Here's how the part is built. I have some questions about the finished solid (model axes, mm). A direction names the side the tool comes from. Give positions to 0.01 mm unless a question says otherwise; leave off trailing zeros. Write each loop counter-clockwise with the first axis right and the second up, starting at its lowest first coordinate (ties: lowest second). Pieces come first, ordered by that corner, then holes. Notation, with made-up numbers: (-6.5, 71) -> (10.5, 71) arc R11 cw to (10.5, 84) -> close; hole circle Ø11 at (9, -4.75). An arc over 180 degrees is marked (long way). Use CSV: the item, a comma, the result in double quotes. Start each with the question number.
(1) If we mould it in two halves opening along X, with no side actions, what happens to faces 1 (the flat face through (-1.5, 4.166, -1.5)), 2 (the flat face through (0, 2, -1.786)), 3 (the cylindrical face through (1.987, -6.439, 0.626))? For each: pulls with the +X half, pulls with the -X half, needs draft (parallel to the pull), parting line crosses it, or undercut.
(2) I need wall thicknesses on L1, parallel to Z at x = 0, y = 2; L2, parallel to Y at x = -2, z = -2.25; L3, parallel to X at y = 1, z = -0.5. Which ranges of each line are inside material? Lowest first, please. Write a range as [from, to].
(3) Suppose I cut it at D-D on y = -1.75. List the corners of the cut face in (x, z) for me.
(4) Suppose I cut it at C-C on x = 0. List the corners of the cut face in (y, z) for me, plus the area to 3 significant figures.
(5) For pin 1 Ø4 at (x, z) = (0.5, 1.5) entering from +Y; pin 2 Ø1 at (y, z) = (-9.5, 1) entering from -X; pin 3 Ø1.8 at (x, z) = (-0.5, 0) entering from +Y; pin 4 Ø1 at (x, y) = (-0.5, -3) entering from +Z, each with a flat end and sliding along its axis, tell me the tip position at first contact or that it passes through.
(6) Suppose I cut it at B-B on z = -1.25. List the corners of the cut face in (x, y) for me.
(7) Suppose I cut it at A-A on y = 2.25. List the corners of the cut face in (x, z) for me.
(8) Which directions (+Z, -Z, +X, -X, +Y, -Y) give clear straight access to the entire face, cutting with the end or side of a thin tool? Please do faces 4 (the flat face through (-0.05, 0, -2.24)), 5 (the cylindrical face through (-0.74, 2.05, -3.35)), 6 (the flat face through (-1.554, 2.405, 0.88)).
from build123d import *

# Parameters (mm, degrees)
CUT_EXTRUDE1_DEPTH = 3.571875


with BuildPart() as part:
    # profiile → Base-Revolve (revolve)
    with BuildSketch(Plane.XY):
        Polygon((0, 4.1656), (3.429, 4.1656), (3.429, 0), (2.0828, 0), (2.0828, -12.7), (0, -12.7), align=None)
    revolve(axis=Axis((0, 9.907210965, 0), (0, -1, 0)))

    # Sketch1 → Cut-Extrude1 (cut)
    with BuildSketch(Plane(origin=(0, 4.1656, 0), x_dir=(1, 0, 0), z_dir=(0, 1, 0))):
        Polygon((2.062222993, 0), (1.031111496, 1.7859375), (-1.031111496, 1.7859375), (-2.062222993, 0), (-1.031111496, -1.7859375), (1.031111496, -1.7859375), align=None)
    extrude(amount=-CUT_EXTRUDE1_DEPTH, mode=Mode.SUBTRACT)


solid = part.part
Geometry says:
1,face 1,"needs draft"
1,face 2,"undercut"
1,face 3,"parting line crosses it"
2,L1,"[-3.43, -1.79], [1.79, 3.43]"
2,L2,"[0, 4.17]"
2,L3,"[-3.39, -1.77], [1.77, 3.39]"
3,outline,"circle Ø4.17 at (0, 0)"
4,outline,"(-12.7, -2.08) -> (0, -2.08) -> (0, -3.43) -> (4.17, -3.43) -> (4.17, -1.79) -> (0.59, -1.79) -> (0.59, 1.79) -> (4.17, 1.79) -> (4.17, 3.43) -> (0, 3.43) -> (0, 2.08) -> (-12.7, 2.08) -> close"
4,area,"68.7 mm²"
5,pin 1,"y = 4.17"
5,pin 2,"x = -2.02"
5,pin 3,"y = 0.59"
5,pin 4,"z = 2.08"
6,outline,"(-3.19, 0) -> (-1.67, 0) -> (-1.67, -12.7) -> (1.67, -12.7) -> (1.67, 0) -> (3.19, 0) -> (3.19, 4.17) -> (1.34, 4.17) -> (1.34, 0.59) -> (-1.34, 0.59) -> (-1.34, 4.17) -> (-3.19, 4.17) -> close"
7,outline,"circle Ø6.86 at (0, 0); hole (-2.06, 0) -> (-1.03, -1.79) -> (1.03, -1.79) -> (2.06, 0) -> (1.03, 1.79) -> (-1.03, 1.79) -> close"
8,face 4,"-Y"
8,face 5,"+Y, -Y"
8,face 6,"+Y"
